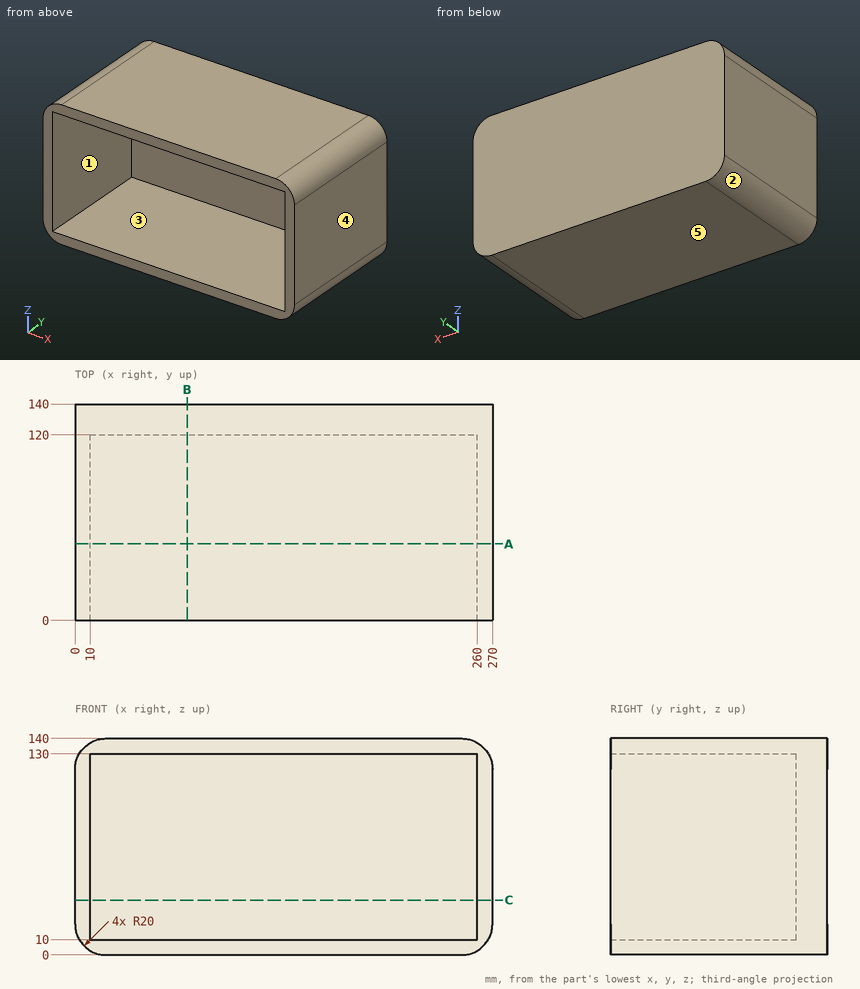
Design review of the part shown in the three views and the two pictorial views. Dimensions are in mm from the part's minimum x, y and z. A direction names the side the tool comes from. Round coordinates to 2 decimals unless told otherwise and drop trailing zeros. Loops run counter-clockwise (first coordinate to the right, second up) from the corner with the lowest first, then second, coordinate; pieces in that order, holes last. Notation, with made-up numbers: M 32,72.5 L 52,72.5 A31 ccw 52,97.5 Z; hole C 66,53.5 d4. An arc over 180 degrees is marked long. Answer as a JSON object with one key per item and string values.
Item 1: We need section C-C on z = 35.5. Give the boundary of the cut face in (x, y), and give its area (3 significant figures).
Answer sheet:
{"outline": "M 0,0 L 10,0 L 10,120 L 260,120 L 260,0 L 270,0 L 270,140 L 0,140 Z", "area": "7,800 mm^2"}
Item 2: Machinability: for the marked faces 1 and 2, which of the approach directions +Z, -Z, +X, -X, +Y, -Y give a long, thin tool a straight path to every point of the face, cutting with its end or side? Answer none if there is none.
Answer sheet:
{"face 1": "-Y", "face 2": "-Z, -X, +Y, -Y"}
Item 3: We need section A-A on y = 49.5. Give the boundary of the cut face in (x, z).
Answer sheet:
{"outline": "M 0,20 A20 ccw 20,0 L 250,0 A20 ccw 270,20 L 270,120 A20 ccw 250,140 L 20,140 A20 ccw 0,120 Z; hole M 10,10 L 260,10 L 260,130 L 10,130 Z"}
Item 4: We need section B-B on x = 72.5. Give the boundary of the cut face in (y, z), and give its area (3 significant figures).
Answer sheet:
{"outline": "M 0,0 L 140,0 L 140,140 L 0,140 L 0,130 L 120,130 L 120,10 L 0,10 Z", "area": "5,200 mm^2"}
Item 5: The part is to be moulded in two halves that separate along X. For the marked faces 3, 4 and 5, say which applies: pulls with the +X half, pulls with the -X half, needs draft (parallel to the pull), parting line crosses it, or undercut.
Answer sheet:
{"face 3": "undercut", "face 4": "pulls with the +X half", "face 5": "needs draft"}
Item 6: Clearance check with flat-ended pins moving along their axes: P1, Ø1.5, axis at x = 224, z = 28.5, coming from the -Y side; P2, Ø2, axis at y = 118.5, z = 17.5, coming from the -X side. State where each tip first meets the part, or that it passes through.
Answer sheet:
{"P1": "stops at y = 120", "P2": "stops at x = 0.06"}
Item 7: Wall thickness on L1, parallel to X at y = 107.5, z = 63; L2, parallel to Z at x = 237.5, y = 14; L3, parallel to Y at x = 257.5, z = 61: over which ranges is each line inside the solid? List them lowest first. Write a range as from..to.
Answer sheet:
{"L1": "x = 0..10, 260..270", "L2": "z = 0..10, 130..140", "L3": "y = 120..140"}
